```python
from build123d import *

# Parameters (mm, degrees)
SKETCH_1_W          = 46
SKETCH_1_H          = 21.3
EXTRUDE_1_DEPTH     = 3
SKETCH_2_R          = 8.3
CUT_EXTRUDE_1_DEPTH = 26.522979842
SKETCH_3_W          = 8
SKETCH_3_H          = 3
CUT_EXTRUDE_2_DEPTH = 26.522979842
SKETCH_4_W          = 5
SKETCH_4_H          = 4
CUT_EXTRUDE_3_DEPTH = 26.522979842
SKETCH_5_W          = 3
SKETCH_5_H          = 2
SKETCH_5_W_2        = 2
SKETCH_5_H_2        = 3
CUT_EXTRUDE_4_DEPTH = 1
HOLE_WIZARD_M3_1_D  = 3.4
SKETCH4_W           = 11
SKETCH4_H           = 2
SKETCH4_W_2         = 13
SKETCH4_H_2         = 3.5
CUT_EXTRUDE3_DEPTH  = 26.522979842
BOSS_EXTRUDE2_DEPTH = 21.3
SKETCH7_W           = 3.011459513
SKETCH7_H           = 21.3
BOSS_EXTRUDE3_DEPTH = 2
SKETCH10_W          = 2
SKETCH10_H          = 28.7
BOSS_EXTRUDE5_DEPTH = 3.011459513
CUT_EXTRUDE6_DEPTH  = 47.808991188
SKETCH14_W          = 16
SKETCH14_H          = 38
BOSS_EXTRUDE8_DEPTH = 3
CHAMFER2_SIZE       = 2
SKETCH15_R          = 1.65
CUT_EXTRUDE7_DEPTH  = 61.720869721
CHAMFER3_SIZE       = 5


with BuildPart() as part:
    # 草圖1 → 填料-伸長1 (new body)
    with BuildSketch(Plane.XY):
        Rectangle(SKETCH_1_W, SKETCH_1_H)
    extrude(amount=EXTRUDE_1_DEPTH)

    # 草圖2 → 除料-伸長1 (cut, through all)
    with BuildSketch(Plane.XY.offset(3)):
        with Locations((-12.7, 0)):
            Circle(SKETCH_2_R)
        with Locations((12.7, 0)):
            Circle(SKETCH_2_R)
    extrude(amount=-CUT_EXTRUDE_1_DEPTH, mode=Mode.SUBTRACT)

    # 草圖3 → 除料-伸長2 (cut, through all)
    with BuildSketch(Plane.XY.offset(3)):
        with Locations((0, 9.15)):
            Rectangle(SKETCH_3_W, SKETCH_3_H)
    extrude(amount=-CUT_EXTRUDE_2_DEPTH, mode=Mode.SUBTRACT)

    # 草圖4 → 除料-伸長3 (cut, through all)
    with BuildSketch(Plane.XY.offset(3)):
        with Locations((0, -5.5)):
            Rectangle(SKETCH_4_W, SKETCH_4_H)
    extrude(amount=-CUT_EXTRUDE_3_DEPTH, mode=Mode.SUBTRACT)

    # 草圖5 → 除料-伸長4 (cut)
    with BuildSketch(Plane.XY.offset(3)):
        with Locations((4, -6.5)):
            Rectangle(SKETCH_5_W, SKETCH_5_H)
        with Locations((-5.5, 8.65)):
            Rectangle(SKETCH_5_W_2, SKETCH_5_H_2)
        with Locations((5.5, 8.65)):
            Rectangle(SKETCH_5_W_2, SKETCH_5_H_2)
        with Locations((-4, -6.5)):
            Rectangle(SKETCH_5_W, SKETCH_5_H)
    extrude(amount=-CUT_EXTRUDE_4_DEPTH, mode=Mode.SUBTRACT)

    # M3 餘隙孔1 (through all)
    with Locations(Plane.XY.offset(3)):
        with Locations((20.35, 8.15), (-20.35, -8.15), (-20.35, 8.15), (20.35, -8.15)):
            Hole(HOLE_WIZARD_M3_1_D / 2)

    # Sketch4 → Cut-Extrude3 (cut, through all)
    with BuildSketch(Plane.XY.offset(3)):
        with Locations((0, -6.5)):
            Rectangle(SKETCH4_W, SKETCH4_H)
        with Locations((0, 8.9)):
            Rectangle(SKETCH4_W_2, SKETCH4_H_2)
    extrude(amount=-CUT_EXTRUDE3_DEPTH, mode=Mode.SUBTRACT)

    # Sketch5 → Boss-Extrude2 (add)
    with BuildSketch(Plane(origin=(0, -10.65, 0), x_dir=(-1, 0, 0), z_dir=(0, -1, 0))):
        Polygon((-23, 0), (-23, -3), (-23.262465991, -3), align=None)
    extrude(amount=-BOSS_EXTRUDE2_DEPTH)

    # Sketch7 → Boss-Extrude3 (add)
    with BuildSketch(Plane(origin=(22.82528916, 0, -1.996954043), x_dir=(-0.08715574274765041, 0, -0.9961946980917462), z_dir=(0.9961946980917462, 0, -0.08715574274765041))):
        with Locations((-3.510311839, 0)):
            Rectangle(SKETCH7_W, SKETCH7_H)
    extrude(amount=BOSS_EXTRUDE3_DEPTH)

    # Sketch10 → Boss-Extrude5 (add)
    with BuildSketch(Plane(origin=(0.437176831, 0, 4.996954043), x_dir=(0.9961946980917463, 0, -0.08715574274765044), z_dir=(0.08715574274765044, 0, 0.9961946980917463))):
        with Locations((23.912478056, 25)):
            Rectangle(SKETCH10_W, SKETCH10_H)
    extrude(amount=-BOSS_EXTRUDE5_DEPTH)

    # Sketch12 → Cut-Extrude6 (cut, through all)
    with BuildSketch(Plane(origin=(0.437176831, 0, 4.996954043), x_dir=(0.9961946980917463, 0, -0.08715574274765044), z_dir=(0.08715574274765044, 0, 0.9961946980917463))):
        Polygon((24.912478056, -5.155045161), (22.912478056, -10.65), (24.912478056, -10.65), align=None)
        Polygon((22.912478056, 39.35), (22.912478056, 10.65), (24.912478056, 16.144954839), (24.912478056, 39.35), align=None)
    extrude(amount=-CUT_EXTRUDE6_DEPTH, mode=Mode.SUBTRACT)

    # Sketch14 → Boss-Extrude8 (add)
    with BuildSketch(Plane(origin=(24.817678556, 0, -2.171265529), x_dir=(-0.08715574274765041, 0, -0.9961946980917462), z_dir=(0.9961946980917462, 0, -0.08715574274765041))):
        with Locations((-10.004582083, 13.844954839)):
            Rectangle(SKETCH14_W, SKETCH14_H)
    extrude(amount=BOSS_EXTRUDE8_DEPTH)

    # Chamfer2
    chamfer2_edges = [part.edges().sort_by_distance(p)[0] for p in [
        (25.254855387, 5.494954839, 2.825688515),
    ]]
    chamfer(chamfer2_edges, length=CHAMFER2_SIZE - 0.0001)  # a hair under: the kernel refuses the full size

    # Sketch15 → Cut-Extrude7 (cut, through all)
    with BuildSketch(Plane(origin=(24.817678556, 0, -2.171265529), x_dir=(0.08715574274765048, 0, 0.9961946980917462), z_dir=(-0.9961946980917462, 0, 0.08715574274765048))):
        with Locations((14.004582083, 25.844954839)):
            Circle(SKETCH15_R)
        with Locations((14.004582083, 1.844954839)):
            Circle(SKETCH15_R)
    extrude(amount=-CUT_EXTRUDE7_DEPTH, mode=Mode.SUBTRACT)

    # Chamfer3
    chamfer3_edges = [part.edges().sort_by_distance(p)[0] for p in [
        (26.486681443, 32.844954839, -0.3050451),
        (27.881173327, 32.844954839, 15.63407007),
        (27.881173327, -5.155045161, 15.63407007),
    ]]
    chamfer(chamfer3_edges, length=CHAMFER3_SIZE)


solid = part.part
```
The model under review builds one solid part; all positions refer to its coordinate system, in mm. A direction names the side the tool comes from. Round coordinates to 2 decimals unless told otherwise and drop trailing zeros. Order: outer loops, then holes, each group sorted by start corner. A loop starts at its lowest first (then second) coordinate and runs counter-clockwise, first axis right, second up.
Item 1: Add section A-A, the plane x = -12.7. State the section outline as (y, z) points, and give its area (3 significant figures).
Working result:
outline: (-10.65, 0) - (-8.3, 0) - (-8.3, 3) - (-10.65, 3) - close; (8.3, 0) - (10.65, 0) - (10.65, 3) - (8.3, 3) - close
area: 14.1 mm2
Item 2: To check wall thickness, follow probe 1 along Y at (x, z) = (20.35, 2.4); probe 2 along Y at (x, z) = (-12.7, 0.7); probe 3 along X at (y, z) = (-5, 1). State the ranges of each line that lie inside material, in increasing order.
Working result:
probe 1: y = -10.65 to -9.85, -6.45 to -3.22, 3.22 to 6.45, 9.85 to 10.65
probe 2: y = -10.65 to -8.3, 8.3 to 10.65
probe 3: x = -23 to -19.32, -6.08 to -2.5, 2.5 to 6.08, 19.32 to 28.11
Item 3: For pin 1 (2.5 mm diameter, centred on y = 8.5, z = 2, fed in from +X); pin 2 (12 mm diameter, centred on x = -16.5, y = 2.5, fed in from -Z); pin 3 (3 mm diameter, centred on x = -20.35, y = -8.15, fed in from -Z); pin 4 (3.5 mm diameter, centred on x = 2, z = 1, fed in from +Y), all flat-tipped, find the tip position at first contact; note any pin that passes through.
Working result:
pin 1: stops at x = 28.3
pin 2: stops at z = 0
pin 3: passes through
pin 4: stops at y = 7.15
Item 4: Draft analysis for pull direction X (two halves, no side actions). For faces 1 (the cylindrical face through (-18.65, -8.08, 1.48)), 2 (the flat face through (-23, 0, 1)), 3 (the flat face through (15, 10.65, 2)), state which applies: released by +X, released by -X, zero draft, split by the parting line, or undercut.
Working result:
face 1: undercut
face 2: released by -X
face 3: zero draft
Item 5: Add section C-C, the plane y = 5. Count the separate pieces of the cut face and the enclosed holes in it, and give its area (3 significant figures).
Working result:
separate pieces: 3
enclosed holes: 0
area: 115 mm2
Item 6: Machinability: for faces 4 (the flat face through (0, -1, 3)), 5 (the flat face through (0, 7.15, 2)), 6 (the flat face through (-2.5, -5, 2)), 7 (the flat face through (26.69, 30.38, 2.22)), which of the approach directions +Z, -Z, +X, -X, +Y, -Y give a long, thin tool a straight path to every point of the face, cutting with its end or side? Answer none if there is none.
Working result:
face 4: +Z, -X, +Y, -Y
face 5: +Z, -Z, +Y
face 6: +Z, -Z
face 7: -Z, -X, +Y
Item 7: Add section D-D, the plane x = 9. State the section outline as (y, z) points.
Working result:
outline: (-10.65, 0) - (-7.43, 0) - (-7.43, 3) - (-10.65, 3) - close; (7.43, 0) - (10.65, 0) - (10.65, 3) - (7.43, 3) - close
Item 8: Add section B-B, the plane x = -20.35. State the section outline as (y, z) points.
Working result:
outline: (-10.65, 0) - (-9.85, 0) - (-9.85, 3) - (-10.65, 3) - close; (-6.45, 0) - (-3.22, 0) - (-3.22, 3) - (-6.45, 3) - close; (3.22, 0) - (6.45, 0) - (6.45, 3) - (3.22, 3) - close; (9.85, 0) - (10.65, 0) - (10.65, 3) - (9.85, 3) - close
